Could you check a few things on this drawing? It's one solid part, dimensions in mm from its lowest x, y, z. Give positions to 0.01 mm unless a question says otherwise; leave off trailing zeros. Loops run counter-clockwise (first coordinate to the right, second up) from the corner with the lowest first, then second, coordinate; pieces in that order, holes last.
1. Imagine slicing it at A-A (z = 63.5). List the corners of the cut face in (x, y) for me (3 decimals).
2. Imagine slicing it at D-D (y = 2.15). Count the separate pieces of the cut face and the enclosed holes in it, plus the area to 3 significant figures.
3. Imagine slicing it at C-C (z = 15.24). List the corners of the cut face in (x, y) for me (3 decimals), plus the area to 3 significant figures.
4. I need wall thicknesses on line 1 along X through (y, z) = (0.9, 15); line 2 along Z through (x, y) = (38.1, 1.3) (3 decimals); line 3 along X through (y, z) = (2.3, 92). Which ranges of each line are inside material? Lowest first, please.
5. Imagine slicing it at B-B (x = 19.05). List the corners of the cut face in (y, z) for me (3 decimals).
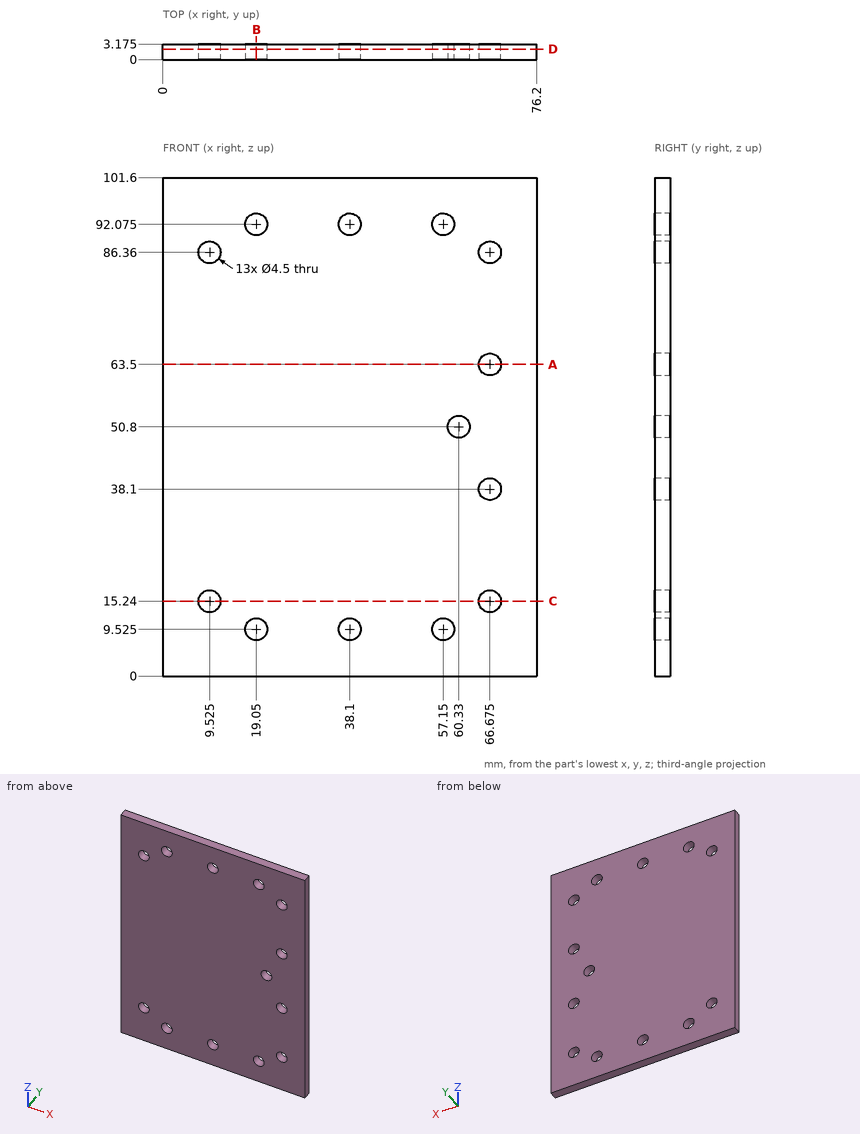
Derived:
1. outline: (0, 0) - (64.425, 0) - (64.425, 3.175) - (0, 3.175) - close; (68.925, 0) - (76.2, 0) - (76.2, 3.175) - (68.925, 3.175) - close
2. separate pieces: 1
2. enclosed holes: 13
2. area: 7,540 mm2
3. outline: (0, 0) - (7.275, 0) - (7.275, 3.175) - (0, 3.175) - close; (11.775, 0) - (64.425, 0) - (64.425, 3.175) - (11.775, 3.175) - close; (68.925, 0) - (76.2, 0) - (76.2, 3.175) - (68.925, 3.175) - close
3. area: 213 mm2
4. line 1: x = 0 to 7.29, 11.76 to 64.44, 68.91 to 76.2
4. line 2: z = 0 to 7.275, 11.775 to 89.825, 94.325 to 101.6
4. line 3: x = 0 to 16.8, 21.3 to 35.85, 40.35 to 54.9, 59.4 to 76.2
5. outline: (0, 0) - (3.175, 0) - (3.175, 7.275) - (0, 7.275) - close; (0, 11.775) - (3.175, 11.775) - (3.175, 89.825) - (0, 89.825) - close; (0, 94.325) - (3.175, 94.325) - (3.175, 101.6) - (0, 101.6) - close
